Model file for the job. Use its own axes, mm. Give positions to 0.01 mm unless a question says otherwise; leave off trailing zeros. Loops run counter-clockwise (first coordinate to the right, second up) from the corner with the lowest first, then second, coordinate; pieces in that order, holes last. Notation, with made-up numbers: M -31.5,40.25 L 2.5,40.25 A26 cw 2.5,70.25 Z; hole C 72,-29 d11. An arc over 180 degrees is marked long. Answer in a Markdown table with one row per item.
Autodesk Inventor part; units mm, degrees
ref_plane "Work Plane2" through (-75, 10, 210) normal (0, 0, 1) x (1, 0, 0)
ref_plane "YZ Plane" through (0, 0, 0) normal (1, 0, 0) x (0, 1, 0)
ref_plane "XZ Plane" through (0, 0, 0) normal (0, 1, 0) x (-1, 0, 0)
sketch "Sketch1" plane through (0, 0, 0) normal (0, 1, 0) x (-1, 0, 0)
  line L0 (-75, 0) -> (75, 0)
  line L1 (75, 0) -> (75, 275)
  line L2 (75, 275) -> (-75, 275) construction
  line L3 (-75, 275) -> (-75, 0)
  circle A0 centre (0, 325) radius 37.5
  line L4 (-75, 275) -> (-31.8965, 344.7197)
  line L5 (75, 275) -> (31.8965, 344.7197)
  point P0 (0, 0)
  point P1 (0, 0)
  dimension "d2" = 75
  dimension "d3" = 50
extrude "Extrusion1" add sketch "Sketch1" along normal blind 10
sketch "Sketch2" plane through (0, 0, 0) normal (0, -1, 0) x (1, 0, 0)
  arc A0 (31.8965, 344.7197) -> (-31.8965, 344.7197) centre (0, 325) ccw
  point P0 (0, 0)
hole "Hole1" at (0, 0, 325) direction (0, 1, 0) diameter 35 end through all
sketch "Sketch3" plane through (-75, 0, 0) normal (-1, 0, 0) x (0, 0, 1)
  line L0 (11, 10) -> (11, 54)
  line L1 (11, 54) -> (41, 84)
  line L2 (41, 84) -> (159, 84)
  line L3 (159, 84) -> (189, 54)
  line L4 (189, 54) -> (189, 10)
  line L5 (0, 10) -> (275, 10)
  line L6 (189, 10) -> (11, 10)
  dimension "d14" = 135
  dimension "d18" = 11
  dimension "d19" = 74
  dimension "d20" = 30
  dimension "d22" = 178
  dimension "d26" = 21
sketch "Sketch6" plane through (-75, 10, 210) normal (0, 0, 1) x (1, 0, 0)
  line L0 (0, 0) -> (10, 0)
  line L1 (10, 0) -> (10, 25)
  line L2 (10, 25) -> (0, 25)
  line L3 (0, 25) -> (0, 0)
  point P0 (75, -10)
  dimension "d27" = 10
  dimension "d28" = 25
sketch3d "3D Sketch1"
sketch "Sketch7" plane through (0, 10, 0) normal (0, 1, 0) x (1, 0, 0)
  circle A0 centre (0, -325) radius 17.5
  circle A1 centre (0, -325) radius 27.5
  point P0 (0, 0)
  dimension "d31" = 10
sketch "Sketch8" plane through (-75, 35, 210) normal (0, 1, 0) x (1, 0, 0)
  line L0 (0, -65) -> (43.1035, -134.7197)
  arc A0 (43.1035, -134.7197) -> (106.8965, -134.7197) centre (75, -115) ccw
  line L1 (106.8965, -134.7197) -> (150, -65)
  line L2 (150, -65) -> (150, 0)
  line L3 (140, 0) -> (150, 0)
  line L4 (140, -62.1584) -> (140, 0)
  line L5 (98.3907, -129.4611) -> (140, -62.1584)
  arc A1 (51.6093, -129.4611) -> (98.3907, -129.4611) centre (75, -115) ccw
  line L6 (10, -62.1584) -> (51.6093, -129.4611)
  line L7 (10, 0) -> (10, -62.1584)
  line L8 (10, 0) -> (0, 0)
  line L9 (0, 0) -> (0, -65)
  line L10 (140, 0) -> (10, 0)
  circle A2 centre (75, -115) radius 17.5
  point P0 (75, 210)
properties part number "Skid Lifting Plate" material "Steel, Galvanized"
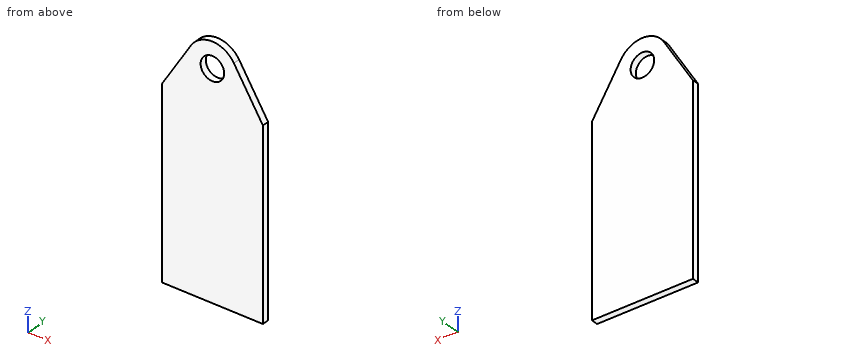
Q1. Saw through at B-B (z = 336). Give the cut face in (x, y).
Reported:
| item | result |
|---|---|
| outline | M -37.29,0 L -13.61,0 L -13.61,10 L -37.29,10 Z; M 13.61,0 L 37.29,0 L 37.29,10 L 13.61,10 Z |
Q2. Saw through at C-C (y = 4.25). Give the cut face in (x, z).
Reported:
| item | result |
|---|---|
| outline | M -75,0 L 75,0 L 75,275 L 31.9,344.72 A37.5 ccw -31.9,344.72 L -75,275 Z; hole C 0,325 d35 |
Q3. Saw through at D-D (x = 42). Give the cut face in (y, z), and give its area (3 significant figures).
Reported:
| item | result |
|---|---|
| outline | M 0,0 L 10,0 L 10,328.38 L 0,328.38 Z |
| area | 3,280 mm² |
Q4. Drop flat-ended pins along their axis: pin 1 (1 mm diameter, centred on x = 21.5, y = 8.5, fed in from +Z); pin 2 (8 mm diameter, centred on x = -22.5, z = 133, fed in from -Y); pin 3 (4 mm diameter, centred on x = -4.5, y = 8.5, fed in from +Z). Give the stop position or say it passes through.
Reported:
| item | result |
|---|---|
| pin 1 | z = 356.07 |
| pin 2 | y = 0 |
| pin 3 | z = 362.42 |
Q5. Saw through at A-A (x = 0). Give the cut face in (y, z).
Reported:
| item | result |
|---|---|
| outline | M 0,0 L 10,0 L 10,307.5 L 0,307.5 Z; M 0,342.5 L 10,342.5 L 10,362.5 L 0,362.5 Z |
Q6. Probe probe 1 along Z at (x, y) = (0, 8.25); probe 2 along X at (y, z) = (3.75, 325); probe 3 along Z at (x, y) = (-2, 9). List the from-to ranges inside material, lowest first.
Reported:
| item | result |
|---|---|
| probe 1 | 0 to 307.5, 342.5 to 362.5 |
| probe 2 | -44.09 to -17.5, 17.5 to 44.09 |
| probe 3 | 0 to 307.61, 342.39 to 362.45 |
